from build123d import *

# Parameters (mm, degrees)
CROQUIS1_W              = 19
CROQUIS1_H              = 40
SALIENTE_EXTRUIR1_DEPTH = 2
REDONDEO1_R             = 1
CROQUIS2_W              = 50.88
CROQUIS2_H              = 2.5
CROQUIS2_W_2            = 1.25
CROQUIS2_H_2            = 7.733481074
SALIENTE_EXTRUIR2_DEPTH = 3
REDONDEO2_R             = 0.75


with BuildPart() as part:
    # Croquis1 → Saliente-Extruir1 (new body)
    with BuildSketch(Plane(origin=(0, 0, 0), x_dir=(1, 0, 0), z_dir=(0, 1, 0))):
        Polygon((26.44, -25), (-26.44, -25), (-26.44, -2), (-29.94, -2), (-29.94, 2), (-26.44, 2), (-26.44, 25), (26.44, 25), (26.44, 2), (29.94, 2), (29.94, -2), (26.44, -2), align=None)
        with Locations((12, -0.5)):
            Rectangle(CROQUIS1_W, CROQUIS1_H, mode=Mode.SUBTRACT)
        with Locations((-12, -0.5)):
            Rectangle(CROQUIS1_W, CROQUIS1_H, mode=Mode.SUBTRACT)
    extrude(amount=SALIENTE_EXTRUIR1_DEPTH)

    # Redondeo1
    redondeo1_edges = [part.edges().sort_by_distance(p)[0] for p in [
        (-26.44, 1, -25),
        (26.44, 1, -25),
        (26.44, 1, 25),
        (-26.44, 1, 25),
    ]]
    fillet(redondeo1_edges, radius=REDONDEO1_R)

    # Croquis2 → Saliente-Extruir2 (add)
    with BuildSketch(Plane(origin=(0, 2, 0), x_dir=(1, 0, 0), z_dir=(0, 1, 0))):
        with Locations((0, 23.75)):
            Rectangle(CROQUIS2_W, CROQUIS2_H)
        with Locations((0, -23.75)):
            Rectangle(CROQUIS2_W, CROQUIS2_H)
        with Locations((-25.815, 0)):
            Rectangle(CROQUIS2_W_2, CROQUIS2_H_2)
        with Locations((25.815, 0)):
            Rectangle(CROQUIS2_W_2, CROQUIS2_H_2)
    extrude(amount=SALIENTE_EXTRUIR2_DEPTH)

    # Redondeo2
    redondeo2_edges = [part.edges().sort_by_distance(p)[0] for p in [
        (0, 5, 22.5),
        (-2.5, 2, 0.5),
        (-12, 2, -19.5),
        (-21.5, 2, 0.5),
        (-12, 2, 20.5),
        (12, 2, 20.5),
        (21.5, 2, 0.5),
        (12, 2, -19.5),
        (2.5, 2, 0.5),
        (0, 5, -22.5),
    ]]
    fillet(redondeo2_edges, radius=REDONDEO2_R)


solid = part.part
Input: part model. Units: mm. Frame: model coordinates. A direction names the side the tool comes from. Coordinates: 2 decimals unless noted, no trailing zeros. Order: outer loops, then holes, each group sorted by start corner. A loop starts at its lowest first (then second) coordinate and runs counter-clockwise, first axis right, second up. Notation, with made-up numbers: M 75,56.25 L 125,56.25 A13 cw 125,70.25 Z; hole C 40,-31 d9. An arc over 180 degrees is marked long. Answer in a Markdown table with one row per item.
(1) Section query A-A, the plane y = 3.15. Output: boundary loops of the cut face in (x, z), plus the area to 3 significant figures.
Numbers:
| item | result |
|---|---|
| outline | M -26.44,-3.87 L -25.19,-3.87 L -25.19,3.87 L -26.44,3.87 Z; M -25.44,-25 L 25.44,-25 L 25.44,-22.5 L -25.44,-22.5 Z; M -25.44,22.5 L 25.44,22.5 L 25.44,25 L -25.44,25 Z; M 25.19,-3.87 L 26.44,-3.87 L 26.44,3.87 L 25.19,3.87 Z |
| area | 274 mm^2 |
(2) Contact query for flat-ended pins moving along their axis: pin 1 Ø6 at (x, z) = (-2.5, -8.5) entering from +Y; pin 2 Ø1.6 at (x, y) = (-28, 1) entering from +Z; pin 3 Ø1.5 at (y, z) = (4, -2) entering from -X. Output: stop coordinate, or through.
Numbers:
| item | result |
|---|---|
| pin 1 | stops at y = 2 |
| pin 2 | stops at z = 2 |
| pin 3 | stops at x = -26.44 |
(3) Section query C-C, the plane z = 3. Output: boundary loops of the cut face in (x, y).
Numbers:
| item | result |
|---|---|
| outline | M -26.44,0 L -21.5,0 L -21.5,1.25 A0.75 ccw -22.25,2 L -25.19,2 L -25.19,5 L -26.44,5 Z; M -2.5,0 L 2.5,0 L 2.5,1.25 A0.75 ccw 1.75,2 L -1.75,2 A0.75 ccw -2.5,1.25 Z; M 21.5,0 L 26.44,0 L 26.44,5 L 25.19,5 L 25.19,2 L 22.25,2 A0.75 ccw 21.5,1.25 Z |
(4) Material intervals for line 1 (X direction, y = 1.35, z = -6.5); line 2 (Z direction, x = 14.5, y = 2.1); line 3 (X direction, y = 4.7, z = -1), sorted ascending. Write a range as [from, to].
Numbers:
| item | result |
|---|---|
| line 1 | x = [-26.44, -21.51], [-2.49, 2.49], [21.51, 26.44] |
| line 2 | z = [-25, -22.5], [22.5, 25] |
| line 3 | x = [-26.44, -25.19], [25.19, 26.44] |
(5) Section query B-B, the plane x = 4. Output: boundary loops of the cut face in (y, z), plus the area to 3 significant figures.
Numbers:
| item | result |
|---|---|
| outline | M 0,-25 L 5,-25 L 5,-23.25 A0.75 ccw 4.25,-22.5 L 2,-22.5 L 2,-20.25 A0.75 ccw 1.25,-19.5 L 0,-19.5 Z; M 0,20.5 L 1.25,20.5 A0.75 ccw 2,21.25 L 2,22.5 L 4.25,22.5 A0.75 ccw 5,23.25 L 5,25 L 0,25 Z |
| area | 34.5 mm^2 |
(6) Draft query along X for faces 5 (the flat face through (2.5, 1, 1)), 6 (the flat face through (25.44, 3, 24)), 7 (the flat face through (0, 2, 25)). Return one class per face: pulls with the +X half, pulls with the -X half, needs draft (parallel to the pull), parting line crosses it, or undercut.
Numbers:
| item | result |
|---|---|
| face 5 | undercut |
| face 6 | pulls with the +X half |
| face 7 | needs draft |
(7) Section query D-D, the plane x = 24. Output: boundary loops of the cut face in (y, z).
Numbers:
| item | result |
|---|---|
| outline | M 0,-25 L 5,-25 L 5,-23.25 A0.75 ccw 4.25,-22.5 L 2,-22.5 L 2,22.5 L 4.25,22.5 A0.75 ccw 5,23.25 L 5,25 L 0,25 Z |
(8) Access query for faces 1 (the flat face through (-28, 2, 0)), 2 (the flat face through (-2.5, 1, 1)), 3 (the flat face through (-25.19, 3, 0)), 4 (the flat face through (28, 1, 2)). Directions: +Z, -Z, +X, -X, +Y, -Y. A direction counts if a zero-diameter tool reaches every point of the face in a straight line with its end or side. Return the directions, or none.
Numbers:
| item | result |
|---|---|
| face 1 | +Z, -Z, -X, +Y |
| face 2 | +Y, -Y |
| face 3 | +Y |
| face 4 | +Z, +X, +Y, -Y |
